Check sheet for the modelled part. Datum: model origin and axes. Units: mm. A direction names the side the tool comes from. Give positions to 0.01 mm unless a question says otherwise; leave off trailing zeros. Order: outer loops, then holes, each group sorted by start corner. A loop starts at its lowest first (then second) coordinate and runs counter-clockwise, first axis right, second up. Notation, with made-up numbers: (7, 71.5) - (43, 71.5) arc R17 ccw to (43, 92.5) - close; hole circle Ø11 at (57.5, 62.25). An arc over 180 degrees is marked (long way). Answer in a Markdown table with one row per item.
from build123d import *

# Parameters (mm, degrees)
F1_DEPTH = 304.8
F2_DEPTH = 2.032
F4_DEPTH = 1.27
F5_DEPTH = 3.175
F6_R     = 3.175


with BuildPart() as f1:
    # F0 (on Right) → F1 (new body)
    with BuildSketch(Plane.YZ):
        Polygon((-2.667, 0), (0, 0), (0, 6.35), (-1.016, 6.35), (-1.016, 0.254), (-1.651, 0.254), (-1.651, 6.35), (-2.667, 6.35), align=None)
    extrude(amount=F1_DEPTH)

    # F2 (add): a face of the model
    f2_faces = [f1.faces().sort_by_distance(p)[0] for p in [
        (152.4, -1.3335, 0),
    ]]
    extrude(f2_faces, amount=F2_DEPTH)

    # F4 (add): a face of the model
    f4_faces = [f1.faces().sort_by_distance(p)[0] for p in [
        (152.4, -2.667, 2.159),
    ]]
    extrude(f4_faces, amount=F4_DEPTH)

    # F3 (on face) → F5 (join)
    with BuildSketch(Plane(origin=(0, 0, -2.032), x_dir=(1, 0, 0), z_dir=(0, 0, -1))):
        with BuildLine():
            Line((136.525, 2.667), (168.275, 2.667))
            ThreePointArc((168.275, 2.667), (152.4, 18.542), (136.525, 2.667))
        make_face()
    extrude(amount=-F5_DEPTH)

    # F6
    f6_edges = [f1.edges().sort_by_distance(p)[0] for p in [
        (152.4, -3.937, 1.143),
        (136.575882, -3.937, -0.4445),
        (168.224118, -3.937, -0.4445),
    ]]
    fillet(f6_edges, radius=F6_R)


solid = f1.part
(1) Mould release check, pull along Y, two halves, no side actions. Record for faces 1 (the flat face through (152, -3, -2.032)), 2 (the flat face through (150, -1.651, 3)), 3 (the flat face through (150, 0, 2)), 4 (the flat face through (150, -3.937, 5)): pulls with the +Y half, pulls with the -Y half, needs draft (parallel to the pull), parting line crosses it, or undercut.
Geometry says:
| item | result |
|---|---|
| face 1 | needs draft |
| face 2 | undercut |
| face 3 | pulls with the +Y half |
| face 4 | pulls with the -Y half |
(2) Thickness scan on L1, parallel to Y at x = 186.5, z = 5; L2, parallel to Z at x = 109, y = -1.5; L3, parallel to Y at x = 284.5, z = -0.75. Record the ranges inside material, lowest first.
Geometry says:
| item | result |
|---|---|
| L1 | -3.94 to -1.65, -1.02 to 0 |
| L2 | -2.03 to 0.25 |
| L3 | -3.94 to 0 |
(3) Cross-section at C-C, the plane x = 161.5. Record the cut outline in (y, z) (3 decimals), then the cut area to 3 significant figures.
Geometry says:
| item | result |
|---|---|
| outline | (-15.675, -2.032) - (0, -2.032) - (0, 6.35) - (-1.016, 6.35) - (-1.016, 0.254) - (-1.651, 0.254) - (-1.651, 6.35) - (-3.937, 6.35) - (-3.937, 4.318) arc R3.175 cw to (-7.112, 1.143) - (-15.675, 1.143) - close |
| area | 68.6 mm² |
(4) Cross-section at B-B, the plane y = -11.5. Record the cut outline in (x, z), then the cut area to 3 significant figures.
Geometry says:
| item | result |
|---|---|
| outline | (139.21, -2.03) - (165.59, -2.03) - (165.59, 1.14) - (139.21, 1.14) - close |
| area | 83.8 mm² |
(5) Cross-section at A-A, the plane x = 282.5. Record the cut outline in (y, z).
Geometry says:
| item | result |
|---|---|
| outline | (-3.94, -2.03) - (0, -2.03) - (0, 6.35) - (-1.02, 6.35) - (-1.02, 0.25) - (-1.65, 0.25) - (-1.65, 6.35) - (-3.94, 6.35) - close |
(6) Gauge pin test, flat ends, axial feed: P1, Ø2, axis at y = -8, z = 1.5, coming from the -X side; P2, Ø3, axis at y = -12.5, z = 4.5, coming from the -X side; P3, Ø5, axis at x = 162, z = 4, coming from the -Y side; P4, Ø9, axis at x = 157.5, y = -14.5, coming from the +Z side. Record the tip position at first contact, or that the pin passes through.
Geometry says:
| item | result |
|---|---|
| P1 | x = 137.15 |
| P2 | through |
| P3 | y = -5.65 |
| P4 | z = 1.14 |
(7) Access from +Z, -Z, +X, -X, +Y, -Y to the whole of each face (thin tool, end or side, straight path). Record for faces 5 (the cylindrical face through (152.7, -18.54, -0.42)), 6 (the flat face through (152, -12, 1.143)), 7 (the flat face through (150, -1.016, 3)).
Geometry says:
| item | result |
|---|---|
| face 5 | +Z, -Z, -Y |
| face 6 | +Z, +X, -X, -Y |
| face 7 | +Z, +X, -X |
